Geometry check sheet. Reference: drawing and pictorial views, mm from the part's lowest x, y, z. A direction names the side the tool comes from. Give positions to 0.01 mm unless a question says otherwise; leave off trailing zeros. Write each loop counter-clockwise with the first axis right and the second up, starting at its lowest first coordinate (ties: lowest second). Pieces come first, ordered by that corner, then holes. Notation, with made-up numbers: M -27,39.5 L 28,39.5 A24 ccw 28,57.5 Z; hole C -11.75,-31 d6. An arc over 180 degrees is marked long. One line per item, written item: value. Start each with the question number.
1. Cross-section at C-C on z = 13. Record the cut outline in (x, y).
2. Gauge pin test, flat ends, axial feed: pin 1 (10 mm diameter, centred on x = 38.5, y = 14, fed in from -Z); pin 2 (5 mm diameter, centred on y = 31.5, z = 7.5, fed in from +X); pin 3 (8 mm diameter, centred on x = 49.5, z = 12.5, fed in from +Y); pin 4 (4 mm diameter, centred on y = 34.5, z = 5.5, fed in from -X). Record the tip position at first contact, or that the pin passes through.
3. Release check for a two-part mould opening along X. For the marked faces 4, 5 and 6 record: pulls with the +X half, pulls with the -X half, needs draft (parallel to the pull), parting line crosses it, or undercut.
4. Cross-section at A-A on x = 5. Record the cut outline in (y, z), then the cut area to 3 significant figures.
5. Tool access check on the marked faces 1, 2 and 3. Record the directions out of +Z, -Z, +X, -X, +Y, -Y that give a thin tool (end or side, any length) a straight path to the whole face; none if there is none.
6. Scan lines: line 1 (X direction, y = 3.85, z = 4); line 2 (Y direction, x = 27.5, z = 7); line 3 (Z direction, x = 50, y = 3.5). Record each from-to range of solid material in increasing order.
7. Cross-section at B-B on x = 27.5. Record the cut outline in (y, z), then the cut area to 3 significant figures.
8. Cross-section at D-D on y = 23. Record the cut outline in (x, z).
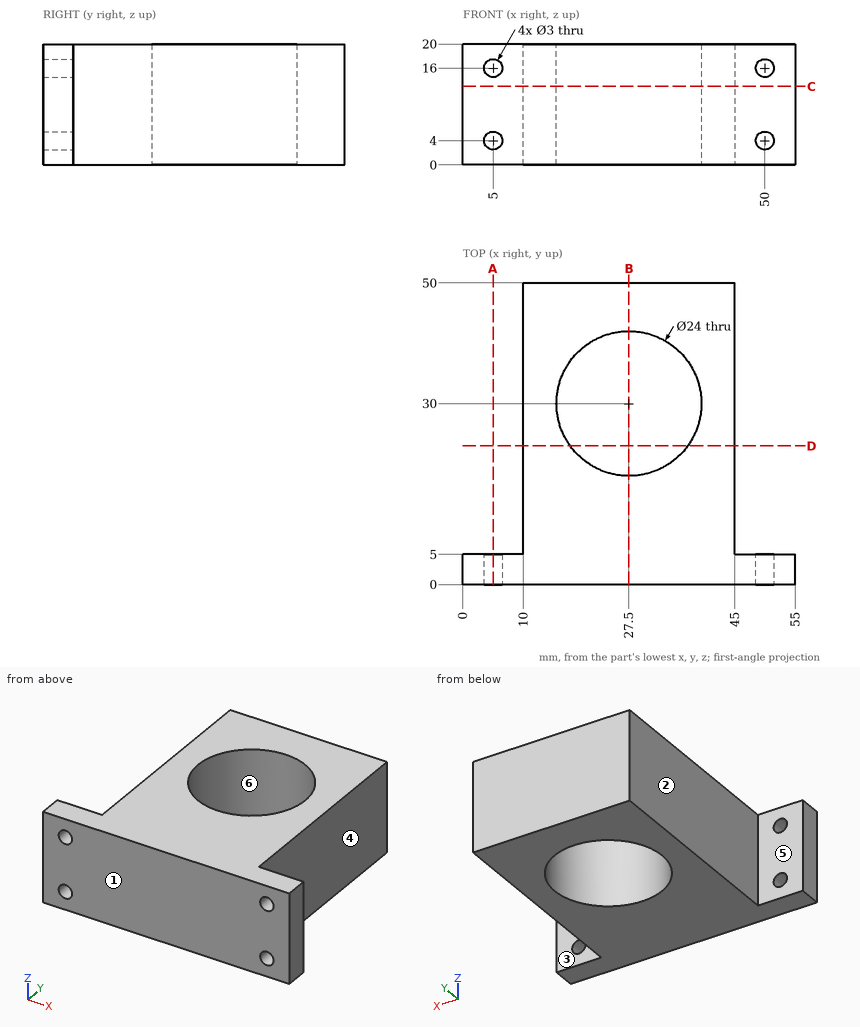
Report:
1. outline: M 0,0 L 55,0 L 55,5 L 45,5 L 45,50 L 10,50 L 10,5 L 0,5 Z; hole C 27.5,30 d24
2. pin 1: stops at z = 0
2. pin 2: stops at x = 45
2. pin 3: stops at y = 5
2. pin 4: stops at x = 10
3. face 4: pulls with the +X half
3. face 5: needs draft
3. face 6: undercut
4. outline: M 0,0 L 5,0 L 5,2.5 L 0,2.5 Z; M 0,5.5 L 5,5.5 L 5,14.5 L 0,14.5 Z; M 0,17.5 L 5,17.5 L 5,20 L 0,20 Z
4. area: 70.0 mm^2
5. face 1: +Z, -Z, +X, -X, -Y
5. face 2: +Z, -Z, -X, +Y
5. face 3: +Z, -Z, +X, +Y
6. line 1: x = 0 to 3.5, 6.5 to 48.5, 51.5 to 55
6. line 2: y = 0 to 18, 42 to 50
6. line 3: z = 0 to 2.5, 5.5 to 14.5, 17.5 to 20
7. outline: M 0,0 L 18,0 L 18,20 L 0,20 Z; M 42,0 L 50,0 L 50,20 L 42,20 Z
7. area: 520 mm^2
8. outline: M 10,0 L 17.75,0 L 17.75,20 L 10,20 Z; M 37.25,0 L 45,0 L 45,20 L 37.25,20 Z
